Geometry check sheet. Reference: the model listing, model coordinates, mm. A direction names the side the tool comes from. Coordinates: 2 decimals unless noted, no trailing zeros. Order: outer loops, then holes, each group sorted by start corner. A loop starts at its lowest first (then second) coordinate and runs counter-clockwise, first axis right, second up. Notation, with made-up numbers: (45, 33) - (51, 33) arc R5 cw to (51, 40) - close; hole circle Ø3 at (-9.5, 63). An arc over 180 degrees is marked (long way). Put each result on its own line as item: value.
from build123d import *

# Parameters (mm, degrees)
SKETCH_1_R          = 1.15
EXTRUDE_1_DEPTH     = 4
SKETCH_2_R          = 3
EXTRUDE_2_DEPTH     = 8
CHAMFER_1_SIZE      = 0.5
CUT_EXTRUDE_START   = -2
CUT_EXTRUDE_2_DEPTH = 2
FILLET_1_R          = 1.2


with BuildPart() as part:
    # 草图1 → 凸台-拉伸1 (new body)
    with BuildSketch(Plane(origin=(0, 0, 0), x_dir=(1, 0, 0), z_dir=(0, 1, 0))):
        with BuildLine():
            ThreePointArc((-6.363461011, -6.362461011), (0, -8.998), (6.363461011, -6.362461011))
            ThreePointArc((6.363461011, -6.362461011), (8.314051085, -3.442824248), (8.999, 0.001))
            ThreePointArc((8.999, 0.001), (8.314051085, 3.444824248), (6.363461011, 6.364461011))
            ThreePointArc((6.363461011, 6.364461011), (0, 9), (-6.363461011, 6.364461011))
            ThreePointArc((-6.363461011, 6.364461011), (-8.999, 0.001), (-6.363461011, -6.362461011))
        make_face()
        with Locations(Location((-6, 0, 0), (0, 0, 270))):
            Circle(SKETCH_1_R, mode=Mode.SUBTRACT)
        with Locations(Location((0, -6, 0), (0, 0, 270))):
            Circle(SKETCH_1_R, mode=Mode.SUBTRACT)
        with Locations(Location((6, 0, 0), (0, 0, 270))):
            Circle(SKETCH_1_R, mode=Mode.SUBTRACT)
        with Locations(Location((0, 6, 0), (0, 0, 270))):
            Circle(SKETCH_1_R, mode=Mode.SUBTRACT)
    extrude(amount=EXTRUDE_1_DEPTH)

    # 草图2 → 凸台-拉伸2 (add)
    with BuildSketch(Plane(origin=(0, 4, 0), x_dir=(1, 0, 0), z_dir=(0, 1, 0))):
        with Locations(Location((0, 0, 0), (0, 0, 270))):
            Circle(SKETCH_2_R)
    extrude(amount=EXTRUDE_2_DEPTH)

    # 倒角1
    chamfer_1_edges = [part.edges().sort_by_distance(p)[0] for p in [
        (0, 12, -3),
    ]]
    chamfer(chamfer_1_edges, length=CHAMFER_1_SIZE)

    # 草图4 → 切除-拉伸2 (cut)
    with BuildSketch(Plane(origin=(0, 4, 0), x_dir=(1, 0, 0), z_dir=(0, 1, 0)).offset(CUT_EXTRUDE_START)):
        with BuildLine():
            Line((5.049644753, 2.094474852), (8.268186553, 3.554868652))
            ThreePointArc((8.268186553, 3.554868652), (8.99927597, -0.114157891), (8.175351882, -3.763458729))
            Line((8.175351882, -3.763458729), (4.91929542, -2.030290031))
            ThreePointArc((4.91929542, -2.030290031), (3.701147604, 0.072647504), (5.049644753, 2.094474852))
        make_face()
        with BuildLine():
            Line((2.094474852, -5.049644753), (3.554868652, -8.268186553))
            ThreePointArc((3.554868652, -8.268186553), (-0.114157891, -8.99927597), (-3.763458729, -8.175351882))
            Line((-3.763458729, -8.175351882), (-2.030290031, -4.91929542))
            ThreePointArc((-2.030290031, -4.91929542), (0.072647504, -3.701147604), (2.094474852, -5.049644753))
        make_face()
        with BuildLine():
            Line((-5.049644753, -2.094474852), (-8.268186553, -3.554868652))
            ThreePointArc((-8.268186553, -3.554868652), (-8.99927597, 0.114157891), (-8.175351882, 3.763458729))
            Line((-8.175351882, 3.763458729), (-4.91929542, 2.030290031))
            ThreePointArc((-4.91929542, 2.030290031), (-3.701147604, -0.072647504), (-5.049644753, -2.094474852))
        make_face()
        with BuildLine():
            Line((-2.094474852, 5.049644753), (-3.554868652, 8.268186553))
            ThreePointArc((-3.554868652, 8.268186553), (0.114157891, 8.99927597), (3.763458729, 8.175351882))
            Line((3.763458729, 8.175351882), (2.030290031, 4.91929542))
            ThreePointArc((2.030290031, 4.91929542), (-0.072647504, 3.701147604), (-2.094474852, 5.049644753))
        make_face()
    extrude(amount=CUT_EXTRUDE_2_DEPTH, mode=Mode.SUBTRACT)

    # 圆角1
    fillet_1_edges = [part.edges().sort_by_distance(p)[0] for p in [
        (-3.762603645, 3, 8.173745459),
        (3.554109286, 3, 8.266512997),
        (-8.174918344, 3, -3.763227961),
        (-8.266990018, 3, 3.554325732),
        (-3.554868652, 3, -8.268186553),
        (3.763458729, 3, -8.175351882),
        (8.174178942, 3, 3.762834384),
        (8.267709465, 3, -3.554652176),
    ]]
    fillet(fillet_1_edges, radius=FILLET_1_R)


solid = part.part
Q1. Thickness scan on L1, parallel to Z at x = 0, y = 1.65; L2, parallel to Y at x = 1.75, z = -6. Record the ranges inside material, lowest first. Write a range as [from, to].
Answer block:
L1: z = [-9, -7.15], [-4.85, 4.85], [7.15, 9]
L2: y = [0, 2]
Q2. Section check B-B on z = 6. Record the boundary of the cut face in (x, y).
Answer block:
outline: (-6.71, 0) - (-1.15, 0) - (-1.15, 2) - (-2.61, 2) - (-2.61, 4) - (-6.71, 4) - close; (1.15, 0) - (6.71, 0) - (6.71, 4) - (2.53, 4) - (2.53, 2) - (1.15, 2) - close
Q3. Section check A-A on x = 0. Record the boundary of the cut face in (y, z), then the cut area to 3 significant figures.
Answer block:
outline: (0, -9) - (2, -9) - (2, -7.15) - (0, -7.15) - close; (0, -4.85) - (2, -4.85) - (2, -3.7) - (4, -3.7) - (4, -3) - (11.5, -3) - (12, -2.5) - (12, 2.5) - (11.5, 3) - (4, 3) - (4, 3.7) - (2, 3.7) - (2, 4.85) - (0, 4.85) - close; (0, 7.15) - (2, 7.15) - (2, 9) - (0, 9) - close
area: 89.3 mm^2
Q4. Access from +Z, -Z, +X, -X, +Y, -Y to the whole of each face (thin tool, end or side, straight path). Record for faces 5 (the cylindrical face through (-3.791, 3.014, -7.773)), 6 (the cylindrical face through (3.7, 3, 0)), 7 (the flat face through (-2.62, 2.99, 6.03)).
Answer block:
face 5: -Z, +Y
face 6: +X, +Y
face 7: +Z, +Y
Q5. Draft check along X on faces 1 (the flat face through (0, 12, 0)), 2 (the flat face through (0, 2, -8)), 3 (the cylindrical face through (0.05, 0.99, 4.85)), 4 (the flat face through (-6.068, 2.986, 2.556)). Enter one of: pulls with the +X half, pulls with the -X half, needs draft (parallel to the pull), parting line crosses it, or undercut.
Answer block:
face 1: needs draft
face 2: undercut
face 3: undercut
face 4: pulls with the -X half
Q6. Section check C-C on x = 6. Record the boundary of the cut face in (y, z), then the cut area to 3 significant figures.
Answer block:
outline: (0, -6.71) - (4, -6.71) - (4, -2.53) - (2, -2.53) - (2, -1.15) - (0, -1.15) - close; (0, 1.15) - (2, 1.15) - (2, 2.61) - (4, 2.61) - (4, 6.71) - (0, 6.71) - close
area: 38.8 mm^2
Q7. Section check D-D on z = -4.25. Record the boundary of the cut face in (x, y), then the cut area to 3 significant figures.
Answer block:
outline: (-7.93, 0) - (7.93, 0) - (7.93, 2) - (7.81, 2) - (7.81, 4) - (1.49, 4) - (1.49, 2) - (-1.49, 2) - (-1.49, 4) - (-7.74, 4) - (-7.74, 2) - (-7.93, 2) - close
area: 56.9 mm^2
Q8. Depth check by flat-ended pin: pin 1 Ø6 at (x, z) = (1, 5.5) entering from +Y; pin 2 Ø4 at (x, z) = (-1, -2.5) entering from -Y; pin 3 Ø4 at (x, y) = (1, 10.5) entering from -Z; pin 4 Ø6 at (x, z) = (7, -2) entering from +Y. Enter the tip coordinate at first touch or a pass-through.
Answer block:
pin 1: stops at y = 11.91
pin 2: stops at y = 0
pin 3: stops at z = -3
pin 4: stops at y = 4
